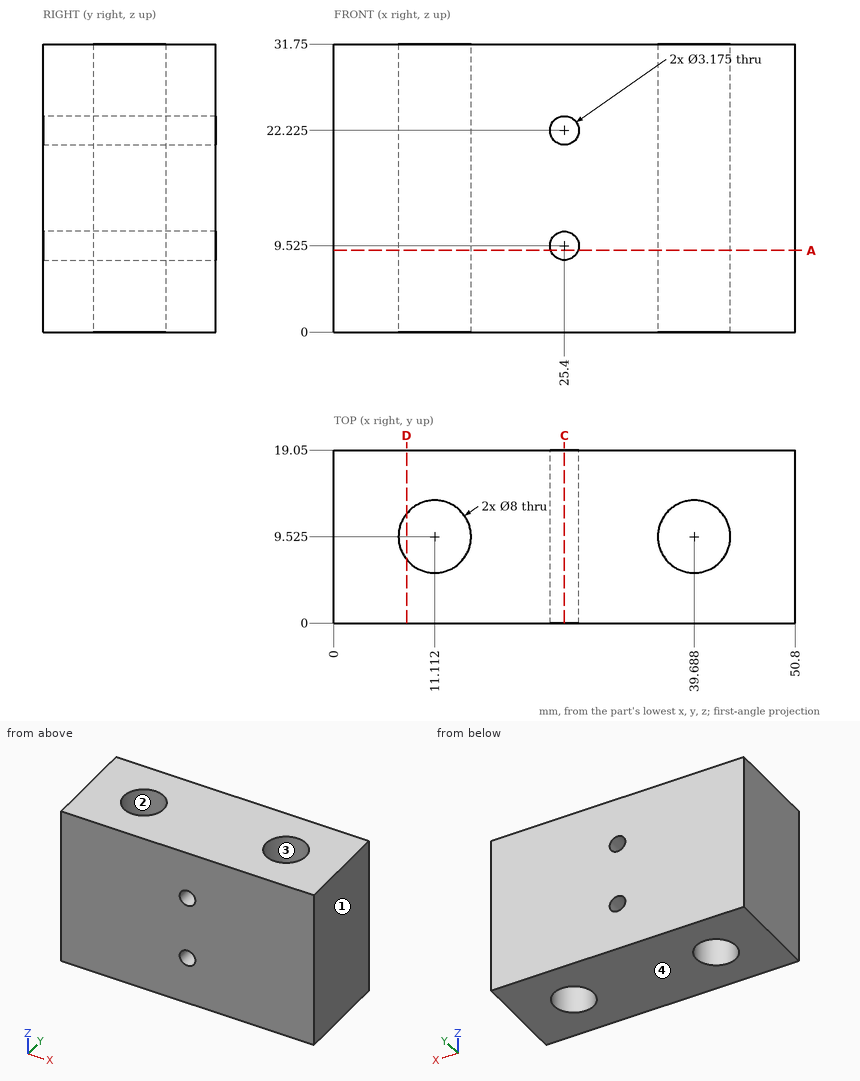
Can you work these out from the drawing? Everything is in mm from the part's minimum corner. Give positions to 0.01 mm unless a question says otherwise; leave off trailing zeros. Order: outer loops, then holes, each group sorted by start corner. A loop starts at its lowest first (then second) coordinate and runs counter-clockwise, first axis right, second up.
1. Suppose I cut it at C-C (x = 25.4). List the corners of the cut face in (y, z) for me, plus the area to 3 significant figures.
2. We'd pull the mould along X, two halves only. Please class the marked faces 1, 2, 3 and 4: pulls with the +X half, pulls with the -X half, needs draft (parallel to the pull), parting line crosses it, or undercut.
3. I need wall thicknesses on L1, parallel to X at y = 7.75, z = 10.5 (1 decimal); L2, parallel to X at y = 10.25, z = 9 (1 decimal); L3, parallel to X at y = 12, z = 4 (1 decimal). Which ranges of each line are inside material? Lowest first, please.
4. Suppose I cut it at A-A (z = 9). Give the number of separate pieces and of enclosed holes in the cut face, plus the area to 3 significant figures.
5. Will this pin go through, and if not, where does the flat tip stop? P1, Ø3, axis at x = 13, y = 9.5, coming from the -Z side.
6. Suppose I cut it at D-D (x = 8). List the corners of the cut face in (y, z) for me.
Solved:
1. outline: (0, 0) - (19.05, 0) - (19.05, 7.94) - (0, 7.94) - close; (0, 11.11) - (19.05, 11.11) - (19.05, 20.64) - (0, 20.64) - close; (0, 23.81) - (19.05, 23.81) - (19.05, 31.75) - (0, 31.75) - close
1. area: 484 mm2
2. face 1: pulls with the +X half
2. face 2: undercut
2. face 3: undercut
2. face 4: needs draft
3. L1: x = 0 to 7.5, 14.7 to 24.1, 26.7 to 36.1, 43.3 to 50.8
3. L2: x = 0 to 7.2, 15 to 23.9, 26.9 to 35.8, 43.6 to 50.8
3. L3: x = 0 to 8, 14.3 to 36.5, 42.8 to 50.8
4. separate pieces: 2
4. enclosed holes: 2
4. area: 810 mm2
5. P1: passes through
6. outline: (0, 0) - (7.01, 0) - (7.01, 31.75) - (0, 31.75) - close; (12.04, 0) - (19.05, 0) - (19.05, 31.75) - (12.04, 31.75) - close
